```python
from build123d import *

# Parameters (mm, degrees)
PAD005_DEPTH    = 45
SKETCH012_R     = 11.2
POCKET006_DEPTH = 15.5210872128
POCKET_DEPTH    = 15.5210872128
POCKET007_DEPTH = 31


with BuildPart() as part:
    # Sketch004 → Pad005 (new body)
    with BuildSketch(Plane.XY):
        Polygon((42, -62), (2, -62), (2, -78.2292272583), (42, -66), align=None)
    extrude(amount=PAD005_DEPTH)

    # Sketch012 → Pocket006 (cut, through all)
    with BuildSketch(Plane(origin=(22.0435767909, -72.1012908672, 0), x_dir=(0.956304756, 0.2923717047, 0), z_dir=(0.2923717047, -0.956304756, 0))):
        with Locations((0, 30)):
            Circle(SKETCH012_R)
    extrude(amount=-POCKET006_DEPTH, mode=Mode.SUBTRACT)

    # Sketch013 → Pocket (cut, through all)
    with BuildSketch(Plane(origin=(22.0435767909, -72.1012908672, 0), x_dir=(0.956304756, 0.2923717047, 0), z_dir=(0.2923717047, -0.956304756, 0))):
        Polygon((0, 56.1345), (33.1881878236, 29.2826289434), (33.1881878236, 69.8913260191), (-31.9570121764, 69.8913260191), (-31.9570121764, 27.8285260191), align=None)
    extrude(amount=-POCKET_DEPTH, mode=Mode.SUBTRACT)

    # Sketch014 → Pocket007 (cut)
    with BuildSketch(Plane.XY.offset(45)):
        Polygon((45.8903901048, -57.7868109147), (-5.585371219, -74.5487714011), (-10.263824653, -60.1813021227), (41.2119366707, -43.4193416363), align=None)
    extrude(amount=-POCKET007_DEPTH, mode=Mode.SUBTRACT)


solid = part.part
```
Model file for the job. Use its own axes, mm. A direction names the side the tool comes from. Coordinates: 2 decimals unless noted, no trailing zeros. Loops run counter-clockwise (first coordinate to the right, second up) from the corner with the lowest first, then second, coordinate; pieces in that order, holes last. Notation, with made-up numbers: (83, 43) - (96, 43) arc R34 ccw to (96, 80) - close; hole circle Ø4 at (19.5, 38). An arc over 180 degrees is marked (long way). Write item = value, one per line. Start each with the question number.
Item 1: Saw through at D-D, the plane z = 32.5. List the corners of the cut face in (x, y).
Item 2: Saw through at B-B, the plane z = 17. List the corners of the cut face in (x, y).
Item 3: Saw through at C-C, the plane x = 34. List the corners of the cut face in (y, z).
Item 4: 3-axis set-ups, long thin cutter, end or side, ignore diameter. For faces 1 (the face through (37.52, -64.83, 42.44)), 2 (the face through (11, -65, 14)): which of +Z, -Z, +X, -X, +Y, -Y reach the whole face in a straight line?
Item 5: Pull direction Z, two halves, no side cores. Call faces 3 (the face through (31.01, -66.04, 25.71)), 4 (the face through (21.72, -72.2, 17.19)), 5 (the face through (17, -68, 0)): +Z half, -Z half, draft (parallel to the pull), parting line (faces both ways), or undercut.
Item 6: Saw through at A-A, the plane z = 25. List the corners of the cut face in (x, y), then the cut area to 3 significant figures.
Item 7: Drop flat-ended pins along their axis: pin 1 Ø2 at (x, z) = (13, 12.5) entering from -Y; pin 2 Ø6 at (x, z) = (11, 21) entering from +Y; pin 3 Ø10 at (x, z) = (10.5, 38.5) entering from +Y. Give the stop position or say it passes through.
Item 8: Wall check: probe 1 along Z at (x, y) = (4.5, -71); probe 2 along Z at (x, y) = (27, -69.5); probe 3 along Z at (x, y) = (22.5, -70.25). Give the ranges that are in metal, low to high. Write a range as [from, to].
Answers:
q1.outline = (2, -78.23) - (11.6, -75.29) - (9.84, -69.53) - (2, -72.08) - close; (30.61, -62.76) - (32.48, -68.91) - (42, -66) - (42, -62) - (32.95, -62) - close
q2.outline = (2, -78.23) - (42, -66) - (42, -62) - (32.95, -62) - (2, -72.08) - close
q3.outline = (-68.45, 0) - (-62, 0) - (-62, 44.49) - (-64.14, 45) - (-68.45, 45) - close
q4.face_1 = +Z, +X, +Y
q4.face_2 = +Z, -X, +Y
q5.face_3 = undercut
q5.face_4 = draft
q5.face_5 = -Z half
q6.outline = (2, -78.23) - (12.46, -75.03) - (10.69, -69.25) - (2, -72.08) - close; (29.75, -63.04) - (31.63, -69.17) - (42, -66) - (42, -62) - (32.95, -62) - close
q6.area = 124 mm2
q7.pin_1 = -75.17
q7.pin_2 = -68.17
q7.pin_3 = -67.75
q8.probe_1 = [0, 14]
q8.probe_2 = [0, 20.24], [39.76, 45]
q8.probe_3 = [0, 18.84], [41.16, 45]
